Part model, mm, in its own coordinate system. A direction names the side the tool comes from. Coordinates: 2 decimals unless noted, no trailing zeros. Order: outer loops, then holes, each group sorted by start corner. A loop starts at its lowest first (then second) coordinate and runs counter-clockwise, first axis right, second up. Notation, with made-up numbers: M -24.5,-20 L -17.5,-20 A8 ccw -17.5,-16 Z; hole C 25,-28 d4. An arc over 180 degrees is marked long. Answer in a Markdown table with one row per item. Add a question column.
from build123d import *

# Parameters (mm, degrees)
F0_W            = 500
F0_H            = 500
F1_DEPTH        = 80
F2_W            = 50
F2_H            = 50
F3_DEPTH        = 500
F3_COPIES_COUNT = 4
F6_DEPTH        = 250
F7_R            = 15


# Not quite as in the source:
# - a pattern or mirror of a feature is missing from the dataset's text; its kind, count and spacing are read off the source's solid


with BuildPart() as f1:
    # F0 (on Top) → F1 (new body)
    with BuildSketch(Plane.XY):
        Rectangle(F0_W, F0_H)
    extrude(amount=F1_DEPTH)

    # F2 (on face) → F3 (join)
    with BuildSketch(Plane(origin=(0, 0, 0), x_dir=(1, 0, 0), z_dir=(0, 0, -1))):
        with Locations((-225, 225)):
            Rectangle(F2_W, F2_H)
    f3 = extrude(amount=F3_DEPTH)

    # F3_copies: F3 ×4 about axis
    f3_copies_axis = Axis((0, 0, 0), (0, 0, 1))
    for i in range(1, F3_COPIES_COUNT):
        add(f3.rotate(f3_copies_axis, i * 360 / F3_COPIES_COUNT))

    # F5 (on Right) → F6 (join, symmetric)
    with BuildSketch(Plane.YZ):
        Polygon((290, 580), (190, 80), (250, 80), (350, 580), align=None)
    extrude(amount=F6_DEPTH, both=True)

    # F7
    f7_edges = [f1.edges().sort_by_distance(p)[0] for p in [
        (0, -250, 80),
        (-250, -30, 80),
        (0, 190, 80),
        (250, -30, 80),
        (-250, 240, 330),
        (250, 240, 330),
        (0, 290, 580),
        (0, 250, 80),
        (-250, 300, 330),
        (0, 350, 580),
        (250, 300, 330),
        (250, 250, -210),
        (-250, 250, -210),
    ]]
    fillet(f7_edges, radius=F7_R)


solid = f1.part
(1) Drop flat-ended pins along their axis: P1, Ø2, axis at x = 90, y = -62.5, coming from the -Z side; P2, Ø5, axis at x = 8, z = 247.5, coming from the -Y side; P3, Ø1.5, axis at x = 103, z = 208, coming from the -Y side. Give the stop position or say it passes through.
(2) Slice it at A-A (z = -374.5). List the corners of the cut face in (x, y).
(3) Slice it at C-C (y = 80). List the corners of the cut face in (x, z).
(4) 3-axis set-ups, long thin cutter, end or side, ignore diameter. For faces 4 (the flat face through (225, 200, -246)), 5 (the flat face through (1, 250, 5)), 6 (the cylindrical face through (245.489, 245.007, 333.225)), 7 (the flat face through (-200, 225, -246)), 8 (the flat face through (-250, -2, 3)): which of +Z, -Z, +X, -X, +Y, -Y reach the whole face in a straight line?
(5) Slice it at B-B (x = 178). List the corners of the cut face in (y, z), and give its area (3 significant figures).
(6) Wall check: line 1 (X direction, y = 216.5, z = -243.5); line 2 (Z direction, x = -101, y = -171.5). Give the ranges that are in metal, low to high.
(7) Pull direction X, two halves, no side cores. Call faces 1 (the cylindrical face through (245.723, 296.093, 333.463)), 2 (the flat face through (200, 225, -246)), 3 (the flat face through (-225, -200, -246)): pulls with the +X half, pulls with the -X half, needs draft (parallel to the pull), parting line crosses it, or undercut.
Computed:
| question | item | result |
|---|---|---|
| 1 | P1 | stops at z = 0 |
| 1 | P2 | stops at y = 223 |
| 1 | P3 | stops at y = 215.45 |
| 2 | outline | M -250,-250 L -200,-250 L -200,-200 L -250,-200 Z; M -250,200 L -200,200 L -200,250 L -235,250 A15 ccw -250,235 Z; M 200,-250 L 250,-250 L 250,-200 L 200,-200 Z; M 200,200 L 250,200 L 250,235 A15 ccw 235,250 L 200,250 Z |
| 3 | outline | M -250,0 L 250,0 L 250,65 A15 ccw 235,80 L -235,80 A15 ccw -250,65 Z |
| 4 | face 4 | -Z, +X, -X |
| 4 | face 5 | -Z, +X, -X, +Y |
| 4 | face 6 | +Z, +X, -Y |
| 4 | face 7 | -Z, +Y, -Y |
| 4 | face 8 | +Z, -Z, -X, +Y, -Y |
| 5 | outline | M -250,0 L 250,0 L 250,78.51 A15 cw 250.29,81.46 L 346.41,562.06 A15 ccw 331.7,580 L 302.3,580 A15 ccw 287.59,567.94 L 192.41,92.06 A15 cw 177.7,80 L -235,80 A15 ccw -250,65 Z |
| 5 | area | 69,900 mm^2 |
| 6 | line 1 | x = -250 to -200, 200 to 250 |
| 6 | line 2 | z = 0 to 80 |
| 7 | face 1 | pulls with the +X half |
| 7 | face 2 | undercut |
| 7 | face 3 | needs draft |
